```python
from build123d import *

# Parameters (mm, degrees)
SKETCH2_W           = 120
SKETCH2_H           = 32
BOSS_EXTRUDE1_DEPTH = 4
SKETCH3_R           = 1.2
SKETCH3_W           = 42
SKETCH3_H           = 21
CUT_EXTRUDE1_DEPTH  = 4
SKETCH4_W           = 60
SKETCH4_H           = 32
BOSS_EXTRUDE2_DEPTH = 4
SKETCH5_R           = 1.2
SKETCH5_W           = 42
SKETCH5_H           = 21
CUT_EXTRUDE2_DEPTH  = 76.153176912
CHAMFER1_SIZE       = 0.5
CHAMFER2_SIZE       = 0.5
CUT_EXTRUDE3_DEPTH  = 10


with BuildPart() as part:
    # Sketch2 → Boss-Extrude1 (new body)
    with BuildSketch(Plane(origin=(0, 0, 0), x_dir=(1, 0, 0), z_dir=(0, 1, 0))):
        Rectangle(SKETCH2_W, SKETCH2_H)
    extrude(amount=BOSS_EXTRUDE1_DEPTH)

    # Sketch3 → Cut-Extrude1 (cut)
    with BuildSketch(Plane(origin=(0, 4, 0), x_dir=(1, 0, 0), z_dir=(0, 1, 0))):
        with Locations(Location((55, 5, 0), (0, 0, 270))):
            Circle(SKETCH3_R)
        with Locations(Location((55, -5, 0), (0, 0, 270))):
            Circle(SKETCH3_R)
        with Locations(Location((5, 5, 0), (0, 0, 270))):
            Circle(SKETCH3_R)
        with Locations(Location((5, -5, 0), (0, 0, 270))):
            Circle(SKETCH3_R)
        with Locations((30, 0)):
            Rectangle(SKETCH3_W, SKETCH3_H)
    extrude(amount=-CUT_EXTRUDE1_DEPTH, mode=Mode.SUBTRACT)

    # Sketch4 → Boss-Extrude2 (add)
    with BuildSketch(Plane.XY.offset(16)):
        with Locations((-30, 16)):
            Rectangle(SKETCH4_W, SKETCH4_H)
    extrude(amount=-BOSS_EXTRUDE2_DEPTH)

    # Sketch5 → Cut-Extrude2 (cut, through all)
    with BuildSketch(Plane.XY.offset(16)):
        with Locations((-5, 21)):
            Circle(SKETCH5_R)
        with Locations((-5, 11)):
            Circle(SKETCH5_R)
        with Locations((-55, 21)):
            Circle(SKETCH5_R)
        with Locations((-55, 11)):
            Circle(SKETCH5_R)
        with Locations((-30, 16)):
            Rectangle(SKETCH5_W, SKETCH5_H)
    extrude(amount=-CUT_EXTRUDE2_DEPTH, mode=Mode.SUBTRACT)

    # Chamfer1
    chamfer1_edges = [part.edges().sort_by_distance(p)[0] for p in [
        (-60, 4, -2),
        (5, 0, 3.8),
        (5, 4, 3.8),
        (5, 0, -6.2),
        (5, 4, -6.2),
        (55, 0, 3.8),
        (55, 4, 3.8),
        (55, 0, -6.2),
        (55, 4, -6.2),
        (51, 0, 0),
        (51, 2, -10.5),
        (30, 0, 10.5),
        (9, 0, 0),
        (9, 2, 10.5),
        (30, 0, -10.5),
        (9, 2, -10.5),
        (51, 4, 0),
        (30, 4, -10.5),
        (9, 4, 0),
        (30, 4, 10.5),
        (60, 4, 0),
        (0, 0, 16),
        (30, 4, 16),
        (-60, 18, 12),
        (-30, 32, 12),
        (-60, 32, 14),
        (0, 4, 14),
        (0, 18, 12),
        (0, 32, 14),
        (-30, 4, 12),
        (0, 18, 16),
        (-30, 32, 16),
        (60, 0, 0),
        (-30, 26.5, 12),
        (-51, 16, 12),
        (-30, 5.5, 12),
        (-9, 16, 12),
        (0, 4, -16),
        (60, 2, 16),
        (-56.2, 11, 12),
        (-56.2, 11, 16),
        (-60, 16, 16),
        (60, 2, -16),
        (-56.2, 21, 12),
        (-56.2, 21, 16),
        (-6.2, 11, 12),
        (-6.2, 11, 16),
        (-6.2, 21, 12),
        (-6.2, 21, 16),
        (-9, 5.5, 14),
        (-51, 5.5, 14),
        (-51, 26.5, 14),
        (-9, 16, 16),
        (-30, 26.5, 16),
        (-51, 16, 16),
        (-30, 5.5, 16),
    ]]
    chamfer(chamfer1_edges, length=CHAMFER1_SIZE)

    # Chamfer2
    chamfer2_edges = [part.edges().sort_by_distance(p)[0] for p in [
        (-0.25, 0, -16),
        (51, 2, 10.5),
        (-60, 1.75, -16),
        (-60, 0, -0.25),
    ]]
    chamfer(chamfer2_edges, length=CHAMFER2_SIZE)

    # Sketch7 → Cut-Extrude3 (cut)
    with BuildSketch(Plane(origin=(0, 4, 0), x_dir=(1, 0, 0), z_dir=(0, 1, 0))):
        Polygon((54.5, 16), (60, 10.5), (63.32506638, 18.331753403), align=None)
        Polygon((54.5, -16), (60, -10.5), (62.093529184, -22.512212848), align=None)
    extrude(amount=-CUT_EXTRUDE3_DEPTH, mode=Mode.SUBTRACT)


solid = part.part
```
Read the model definition and answer for the solid it produces. Units are mm, in the model's axes. A direction names the side the tool comes from. Coordinates: 2 decimals unless noted, no trailing zeros. Write each loop counter-clockwise with the first axis right and the second up, starting at its lowest first coordinate (ties: lowest second). Pieces come first, ordered by that corner, then holes. Notation, with made-up numbers: (69.25, 71.5) - (116.25, 71.5) arc R15 ccw to (116.25, 85.5) - close; hole circle Ø4 at (-7, 47.25). An arc over 180 degrees is marked (long way). Answer as a JSON object with one key per item and string values. Group by question number.
1. A cutting plane is placed at B-B (x = -55). Determine the outline of the cut face in (y, z), plus the area to 3 significant figures.
2. A cutting plane is placed at A-A (y = 11). Give the number of separate pieces and of enclosed holes in the cut face, plus the area to 3 significant figures.
3. Consider L1, parallel to X at y = 1.8, z = -5; L2, parallel to Y at x = -55, z = 14.55; L3, parallel to X at y = 23, z = 13.5. Determine where each line is inside the solid, lowest interval first. Write a range as [from, to].
4. Each of these flat-tipped pins is pushed along its axis until it touches: P1, Ø3, axis at x = -55, y = 11, coming from the +Z side; P2, Ø1.9, axis at x = -5, y = 21, coming from the +Z side; P3, Ø10, axis at x = -47, y = 10.5, coming from the -Z side; P4, Ø3, axis at x = 7.5, z = -8, coming from the -Y side. Where does it stop, or does it pass through?
5. The mould has two halves that part along X. Classify faces 1 (the flat face through (-30, 5.5, 14)), 2 (the flat face through (-30, 32, 14)), 3 (the flat face through (60, 2, 0)): +X half, -X half, draft (parallel to the pull), parting line (faces both ways), or undercut.
6. A cutting plane is placed at D-D (y = 17). Determine the outline of the cut face in (x, z), plus the area to 3 significant figures.
7. Which of the six approach directions +Z, -Z, +X, -X, +Y, -Y give full straight-line access (tool end or side, diameter ignored) to faces 4 (the flat face through (30, 2, -10.5)), 5 (the flat face through (57.2, 2, -13.3)), 6 (the flat face through (-30, 26.5, 14))?
Worked out:
{
 "1": {"outline": "(0, -15.5) - (0.5, -16) - (3.5, -16) - (4, -15.5) - (4, 11.5) - (4.5, 12) - (9.3, 12) - (9.8, 12.5) - (9.8, 15.5) - (9.3, 16) - (0.5, 16) - (0, 15.5) - close; (12.2, 12.5) - (12.7, 12) - (19.3, 12) - (19.8, 12.5) - (19.8, 15.5) - (19.3, 16) - (12.7, 16) - (12.2, 15.5) - close; (22.2, 12.5) - (22.7, 12) - (31.5, 12) - (32, 12.5) - (32, 15.5) - (31.5, 16) - (22.7, 16) - (22.2, 15.5) - close", "area": "219 mm²"},
 "2": {"separate pieces": "4", "enclosed holes": "0", "area": "50.8 mm²"},
 "3": {"L1": "x = [-60, 3.8], [6.2, 9], [51, 53.8], [56.2, 60]", "L2": "y = [0, 9.8], [12.2, 19.8], [22.2, 32]", "L3": "x = [-60, -51], [-9, 0]"},
 "4": {"P1": "stops at z = 15.8", "P2": "passes through", "P3": "stops at z = 12", "P4": "stops at y = 0"},
 "5": {"face 1": "undercut", "face 2": "draft", "face 3": "+X half"},
 "6": {"outline": "(-60, 12.5) - (-59.5, 12) - (-51.5, 12) - (-51, 12.5) - (-51, 15.5) - (-51.5, 16) - (-59.5, 16) - (-60, 15.5) - close; (-9, 12.5) - (-8.5, 12) - (-0.5, 12) - (0, 12.5) - (0, 15.5) - (-0.5, 16) - (-8.5, 16) - (-9, 15.5) - close", "area": "71.0 mm²"},
 "7": {"face 4": "+Y, -Y", "face 5": "-Z, +X, +Y, -Y", "face 6": "+Z, -Z"}
}
